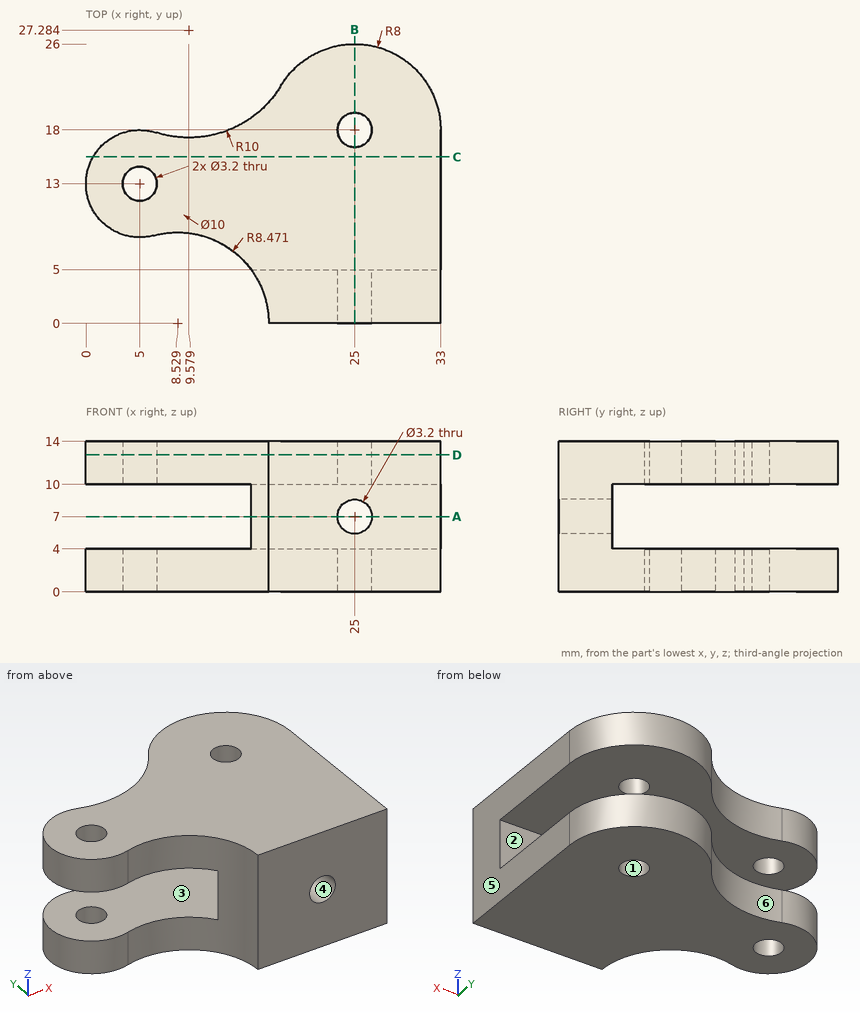
Verification items for this drawing (mm, ordinates from the low corner). A direction names the side the tool comes from. Coordinates: 2 decimals unless noted, no trailing zeros. Loops run counter-clockwise (first coordinate to the right, second up) from the corner with the lowest first, then second, coordinate; pieces in that order, holes last. Notation, with made-up numbers: (0.5, 76.25) -> (50.5, 76.25) arc R12 ccw to (50.5, 93.25) -> close; hole circle Ø10 at (-1, 28). An arc over 180 degrees is marked (long way). Answer in a Markdown table with one row per item. Add a question column.
1. Draft check along X on the marked faces 3, 4, 5 and 6. Enter one of: +X half, -X half, draft (parallel to the pull), parting line (faces both ways), or undercut.
2. Section check C-C, the plane y = 15.5. Enter the section's corners in (x, z).
3. Access from +Z, -Z, +X, -X, +Y, -Y to the whole of each face (thin tool, end or side, straight path). Record for the marked faces 1 and 2.
4. Material ranges on probe 1 along Z at (x, y) = (25, 2.8); probe 2 along Z at (x, y) = (18, 13); probe 3 along Y at (x, z) = (5, 2), recorded low to high. Write a range as [from, to].
5. Section check B-B, the plane x = 25. Enter the section's corners in (y, z).
6. Depth check by flat-ended pin: P1, Ø1.8, axis at x = 28, z = 7, coming from the +Y side; P2, Ø1, axis at x = 20.5, z = 12.5, coming from the +Y side. Enter the tip coordinate at first touch or a pass-through.
7. Section check D-D, the plane z = 12.75. Enter the section's corners in (x, y) (1 decimal).
8. Section check A-A, the plane z = 7. Enter the section's corners in (x, y), then the cut area to 3 significant figures.
Derived:
| question | item | result |
|---|---|---|
| 1 | face 3 | draft |
| 1 | face 4 | undercut |
| 1 | face 5 | +X half |
| 1 | face 6 | undercut |
| 2 | outline | (0.67, 0) -> (33, 0) -> (33, 4) -> (0.67, 4) -> close; (0.67, 10) -> (33, 10) -> (33, 14) -> (0.67, 14) -> close |
| 3 | face 1 | +Z, -Z |
| 3 | face 2 | +X, -X, +Y |
| 4 | probe 1 | z = [0, 5.4], [8.6, 14] |
| 4 | probe 2 | z = [0, 4], [10, 14] |
| 4 | probe 3 | y = [8, 11.4], [14.6, 18] |
| 5 | outline | (0, 0) -> (16.4, 0) -> (16.4, 4) -> (5, 4) -> (5, 5.4) -> (0, 5.4) -> close; (0, 8.6) -> (5, 8.6) -> (5, 10) -> (16.4, 10) -> (16.4, 14) -> (0, 14) -> close; (19.6, 0) -> (26, 0) -> (26, 4) -> (19.6, 4) -> close; (19.6, 10) -> (26, 10) -> (26, 14) -> (19.6, 14) -> close |
| 6 | P1 | stops at y = 5 |
| 6 | P2 | stops at y = 24.93 |
| 7 | outline | (6.3, 8.2) arc R8.5 cw to (17, 0) -> (33, 0) -> (33, 18) arc R8 ccw to (18.1, 22.1) arc R10 cw to (6.5, 17.8) arc R5 ccw (long way) to start; hole circle Ø3.2 at (5, 13); hole circle Ø3.2 at (25, 18) |
| 8 | outline | (15.37, 5) arc R8.47 cw to (17, 0) -> (23.4, 0) -> (23.4, 5) -> close; (26.6, 0) -> (33, 0) -> (33, 5) -> (26.6, 5) -> close |
| 8 | area | 66.6 mm² |
